Work out the finished part from the listing and answer in its coordinate system (mm). A direction names the side the tool comes from. Round coordinates to 2 decimals unless told otherwise and drop trailing zeros. Write each loop counter-clockwise with the first axis right and the second up, starting at its lowest first coordinate (ties: lowest second). Pieces come first, ordered by that corner, then holes. Notation, with made-up numbers: (64, 54) -> (120, 54) arc R22 ccw to (120, 86) -> close; hole circle Ø7 at (-21.75, 28). An arc over 180 degrees is marked (long way). Answer as a JSON object with one key per item and string values. Group by question number.
from build123d import *

# Parameters (mm, degrees)
F1_DEPTH = 76.2
F2_R     = 11.1125
F3_R     = 5.08
F4_W     = 25.4
F4_H     = 9.6059094062
F4_H_2   = 10.5453204632
F5_DEPTH = 25.4
F6_W     = 25.4
F6_H     = 12.6698460698
F6_H_2   = 15.3897032142
F7_DEPTH = 25.4


with BuildPart() as f1:
    # F0 (on Front) → F1 (new body, symmetric)
    with BuildSketch(Plane.XZ):
        with BuildLine():
            ThreePointArc((85.5011615648, -96.0432013591), (0, -128.5875), (-85.5011615648, -96.0432013591))
            ThreePointArc((-85.5011615648, -96.0432013591), (-85.91339025, -95.6746284654), (-86.3240301315, -95.3042862526))
            Line((-86.3240301315, -95.3042862526), (-72.8343228145, -81.8145789356))
            ThreePointArc((-72.8343228145, -81.8145789356), (-75.1761291277, -79.6681461792), (-77.4547090442, -77.4547090442))
            Line((-77.4547090442, -77.4547090442), (-90.9250932258, -90.9250932258))
            Line((-90.9250932258, -90.9250932258), (-95.4152212864, -95.4152212864))
            ThreePointArc((-95.4152212864, -95.4152212864), (0, -134.9375), (95.4152212864, -95.4152212864))
            Line((95.4152212864, -95.4152212864), (77.4547090442, -77.4547090442))
            ThreePointArc((77.4547090442, -77.4547090442), (75.1761291277, -79.6681461792), (72.8343228145, -81.8145789356))
            Line((72.8343228145, -81.8145789356), (86.3240301315, -95.3042862526))
            ThreePointArc((86.3240301315, -95.3042862526), (85.91339025, -95.6746284654), (85.5011615648, -96.0432013591))
        make_face()
    extrude(amount=F1_DEPTH, both=True)

    # F2
    f2_edges = [f1.edges().sort_by_distance(p)[0] for p in [
        (95.415221, 0, -95.415221),
        (-95.415221, 0, -95.415221),
    ]]
    fillet(f2_edges, radius=F2_R)

    # F3
    f3_edges = [f1.edges().sort_by_distance(p)[0] for p in [
        (-86.32403, 0, -95.304286),
        (86.32403, 0, -95.304286),
    ]]
    fillet(f3_edges, radius=F3_R)

    # F4 (on face) → F5 (cut)
    with BuildSketch(Plane(origin=(0, 0, 0), x_dir=(0, 1, 0), z_dir=(0.7071067812, 0, 0.7071067812))):
        with Locations((-44.45, -111.0845452969)):
            Rectangle(F4_W, F4_H)
        with Locations((44.45, -111.0845452969)):
            Rectangle(F4_W, F4_H)
        with Locations((0, -110.6148397684)):
            Rectangle(F4_W, F4_H_2)
    extrude(amount=-F5_DEPTH, mode=Mode.SUBTRACT)

    # F6 (on face) → F7 (cut)
    with BuildSketch(Plane(origin=(0, 0, 0), x_dir=(0, -1, 0), z_dir=(-0.7071067812, 0, 0.7071067812))):
        with Locations((-44.45, -109.5525769651)):
            Rectangle(F6_W, F6_H)
        with Locations((44.45, -109.5525769651)):
            Rectangle(F6_W, F6_H)
        with Locations((0, -108.1926483929)):
            Rectangle(F6_W, F6_H_2)
    extrude(amount=-F7_DEPTH, mode=Mode.SUBTRACT)


solid = f1.part
1) A cutting plane is placed at B-B on x = 10.5. Determine the outline of the cut face in (y, z), plus the area to 3 significant figures.
2) For a pull along X with two mould halves and no side action, classify faces 1 (the face through (-79.73, 44.63, -84.16)), 2 (the face through (90.453, -1.067, -95.432)), 3 (the face through (-77, -57.15, -82)), 4 (the face through (-83, -1, -83)) as released by +X, released by -X, zero draft, split by the parting line, or undercut.
3) A cutting plane is placed at A-A on z = -124.5. Determine the outline of the cut face in (x, y).
4) Straight lines are drawn through the part: L1, parallel to X at y = 0, z = -87; L2, parallel to X at y = 6.5, z = -108; L3, parallel to Z at x = -81, y = 2. For each, find the intervals that lie inside material, in ascending order.
5) A cutting plane is placed at D-D on x = 44. Determine the outline of the cut face in (y, z).
6) A cutting plane is placed at C-C on z = -109.5. Determine the outline of the cut face in (x, y), plus the area to 3 significant figures.
7) Each of these flat-tipped pins is pushed along its axis until it touches: P1, Ø10, axis at y = 2, z = -101, coming from the -X side; P2, Ø5, axis at x = 22.5, y = 43.5, coming from the +Z side; P3, Ø4, axis at x = 14.5, y = -4.5, coming from the +Z side. Where does it stop, or does it pass through?
8) A tool of negligible diameter and unlimited length cuts with its end or side. For faces 5 (the face through (-75.14, -66.81, -79.7)), 6 (the face through (-1.31, -1.07, -134.93)), 7 (the face through (77, -12.7, -82)), from which of +Z, -Z, +X, -X, +Y, -Y can it reach the whole face along a straight path? Write none if from no direction.
Established:
{
 "1": {"outline": "(-76.2, -134.53) -> (76.2, -134.53) -> (76.2, -128.16) -> (-76.2, -128.16) -> close", "area": "971 mm²"},
 "2": {"face 1": "undercut", "face 2": "released by +X", "face 3": "undercut", "face 4": "released by -X"},
 "3": {"outline": "(-52.04, -76.2) -> (-32.16, -76.2) -> (-32.16, 76.2) -> (-52.04, 76.2) -> close; (32.16, -76.2) -> (52.04, -76.2) -> (52.04, 76.2) -> (32.16, 76.2) -> close"},
 "4": {"L1": "x = -87 to -78.02, 78.02 to 87", "L2": "x = -80.9 to -69.79, 69.79 to 80.9", "L3": "z = -107.92 to -99.87, -89.98 to -82.89"},
 "5": {"outline": "(-76.2, -127.56) -> (76.2, -127.56) -> (76.2, -120.83) -> (-76.2, -120.83) -> close"},
 "6": {"outline": "(-78.85, -76.2) -> (-67.41, -76.2) -> (-67.41, 76.2) -> (-78.85, 76.2) -> close; (67.41, -76.2) -> (78.85, -76.2) -> (78.85, 76.2) -> (67.41, 76.2) -> close", "area": "3,490 mm²"},
 "7": {"P1": "stops at x = -90.42", "P2": "stops at z = -126.13", "P3": "stops at z = -127.52"},
 "8": {"face 5": "+Z, +Y, -Y", "face 6": "-Z, +Y, -Y", "face 7": "+Z"}
}
